```python
from build123d import *

# Parameters (mm, degrees)
F1_DEPTH = 20
F2_SIZE  = 0.8
F3_SIZE  = 1


with BuildPart() as f1:
    # F0 (on Top) → F1 (new body)
    with BuildSketch(Plane.XY):
        Polygon((-15, 4.9), (-15, 0), (-13.403978, 0), (-13.403978, 3.3), (13.396022, 3.3), (13.396022, 0), (15, 0), (15, 4.9), align=None)
        Polygon((-13.403978, 0), (-15, 0), (-15, -4.7), (-5, -4.7), (-5, -3.1), (-13.403978, -3.1), (-13.403978, -1.6), (13.396022, -1.600005), (13.399751, -3.1), (5, -3.1), (5, -4.7), (15, -4.7), (15, 0), (13.396022, 0), align=None)
    extrude(amount=F1_DEPTH)

    # F2
    f2_edges = [f1.edges().sort_by_distance(p)[0] for p in [
        (-5, -3.1, 10),
        (5, -3.1, 10),
    ]]
    chamfer(f2_edges, length=F2_SIZE)

    # F3
    f3_edges = [f1.edges().sort_by_distance(p)[0] for p in [
        (-15, 4.9, 10),
        (-15, 0.1, 20),
        (-15, -4.7, 10),
        (-15, 0.1, 0),
        (15, 4.9, 10),
        (15, 0.1, 0),
        (15, -4.7, 10),
        (15, 0.1, 20),
    ]]
    chamfer(f3_edges, length=F3_SIZE)


solid = f1.part
```
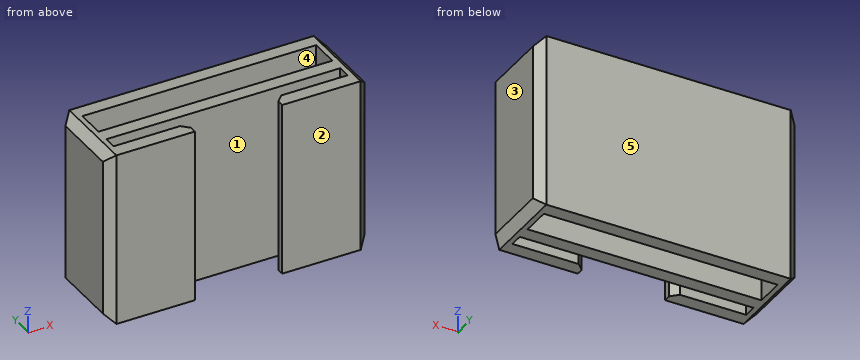
Part model, mm, in its own coordinate system. Face numbers are marked on the shaded views. A direction names the side the tool comes from. Give positions to 0.01 mm unless a question says otherwise; leave off trailing zeros. Loops run counter-clockwise (first coordinate to the right, second up) from the corner with the lowest first, then second, coordinate; pieces in that order, holes last. Notation, with made-up numbers: M 51.25,49.25 L 68.25,49.25 A25 ccw 68.25,82.25 Z; hole C 80.5,19 d1. An arc over 180 degrees is marked long. Return JSON: item names as keys, results as strings.
1) Pull direction Y, two halves, no side cores. Call the marked faces 3, 4 and 5: released by +Y, released by -Y, zero draft, split by the parting line, or undercut.
Calculated:
{"face 3": "zero draft", "face 4": "undercut", "face 5": "released by +Y"}
2) 3-axis set-ups, long thin cutter, end or side, ignore diameter. For the marked faces 1 and 2: which of +Z, -Z, +X, -X, +Y, -Y reach the whole face in a straight line?
Calculated:
{"face 1": "+Z, -Z", "face 2": "+Z, -Z, +X, -X, -Y"}
3) Drill centre lines: line 1 (Y direction, x = 12.5, z = 11.5); line 2 (Y direction, x = 0.5, z = 11.75); line 3 (X direction, y = -2.5, z = 2.75). Where is each one in solid material? Low to high.
Calculated:
{"line 1": "y = -4.7 to -3.1, -1.6 to 0, 3.3 to 4.9", "line 2": "y = -1.6 to 0, 3.3 to 4.9", "line 3": "x = -15 to -13.4, 13.4 to 15"}
4) Saw through at C-C, the plane z = 15.75. List the corners of the cut face in (x, y), then the cut area to 3 significant figures.
Calculated:
{"outline": "M -15,-3.7 L -14,-4.7 L -5,-4.7 L -5,-3.9 L -5.8,-3.1 L -13.4,-3.1 L -13.4,-1.6 L 13.4,-1.6 L 13.4,-3.1 L 5.8,-3.1 L 5,-3.9 L 5,-4.7 L 14,-4.7 L 15,-3.7 L 15,3.9 L 14,4.9 L -14,4.9 L -15,3.9 Z; hole M -13.4,0 L 13.4,0 L 13.4,3.3 L -13.4,3.3 Z", "area": "141 mm2"}
5) Saw through at D-D, the plane x = -0.25. List the corners of the cut face in (y, z), then the cut area to 3 significant figures.
Calculated:
{"outline": "M -1.6,0 L 0,0 L 0,20 L -1.6,20 Z; M 3.3,0 L 4.9,0 L 4.9,20 L 3.3,20 Z", "area": "64.0 mm2"}
6) Saw through at A-A, the plane y = 1. List the corners of the cut face in (x, z), then the cut area to 3 significant figures.
Calculated:
{"outline": "M -15,1 L -14,0 L -13.4,0 L -13.4,20 L -14,20 L -15,19 Z; M 13.4,0 L 14,0 L 15,1 L 15,19 L 14,20 L 13.4,20 Z", "area": "62.0 mm2"}
7) Saw through at B-B, the plane x = -7.5. List the corners of the cut face in (y, z), then the cut area to 3 significant figures.
Calculated:
{"outline": "M -4.7,0 L -3.1,0 L -3.1,20 L -4.7,20 Z; M -1.6,0 L 0,0 L 0,20 L -1.6,20 Z; M 3.3,0 L 4.9,0 L 4.9,20 L 3.3,20 Z", "area": "96.0 mm2"}
